Part model, mm, in its own coordinate system. Face numbers are marked on the shaded views. A direction names the side the tool comes from. Coordinates: 2 decimals unless noted, no trailing zeros. Loops run counter-clockwise (first coordinate to the right, second up) from the corner with the lowest first, then second, coordinate; pieces in that order, holes last.
```python
from build123d import *

# Parameters (mm, degrees)
F0_W     = 20.32
F0_H     = 19.186653
F1_DEPTH = 2.26077
F2_W     = 4.396148
F2_H     = 12.7
F3_DEPTH = 12.18664


with BuildPart() as f1:
    # F0 (on Front) → F1 (new body)
    with BuildSketch(Plane.XZ):
        with Locations((-10.16, 11.454718)):
            Rectangle(F0_W, F0_H)
    extrude(amount=F1_DEPTH)

    # F2 (on face) → F3 (join)
    with BuildSketch(Plane.XZ.offset(2.26077)):
        with Locations((-15.614839, 11.398978)):
            Rectangle(F2_W, F2_H)
        with Locations((-4.54603, 11.398978)):
            Rectangle(F2_W, F2_H)
    extrude(amount=F3_DEPTH)


solid = f1.part
```
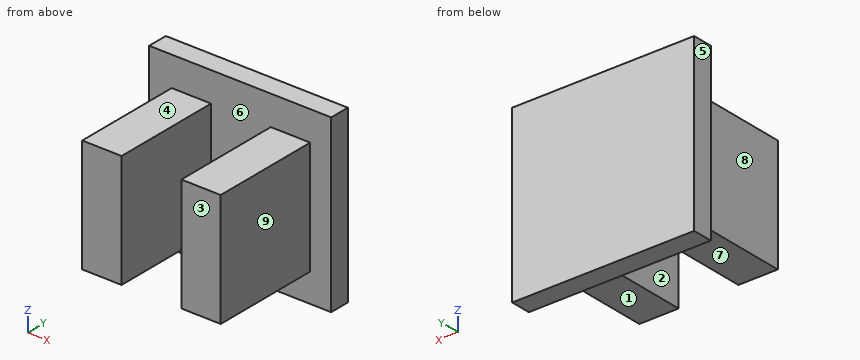
Q1. Tool access for the marked faces 1, 2, 3, 4 and 5: list every direction of +Z, -Z, +X, -X, +Y, -Y with a clear straight run to the whole face (end or side of a thin tool).
Q2. Mould opens along X. For the marked faces 6, 7, 8 and 9 say: released by +X, released by -X, zero draft, split by the parting line, or undercut.
Q3. Saw through at A-A (y = -11.25). List the corners of the cut face in (x, z).
Q4. Saw through at C-C (z = 14.5). List the corners of the cut face in (x, y), plus the area to 3 significant figures.
Q5. Probe line 1 (X direction, y = -12, z = 13.5); line 2 (Y direction, x = -12, z = 12.25); line 3 (Z direction, x = -4.75, y = -7.5). List the from-to ranges inside material, lowest first.
Q6. Saw through at D-D (z = 3.75). List the corners of the cut face in (x, y).
Q7. Saw through at B-B (x = -15.5). List the corners of the cut face in (y, z), plus the area to 3 significant figures.
Q8. Drop flat-ended pins along their axis: P1, Ø10, axis at x = -12, z = 4, coming from the -Y side; P2, Ø5, axis at x = -5, y = -10.5, coming from the -Z side; P3, Ø2, axis at y = -12, z = 7, coming from the +X side; P4, Ø2, axis at x = -16.5, y = -9.5, coming from the +Z side. Give the stop position or say it passes through.
Checked values:
1. face 1: -Z, +X, -X, -Y
1. face 2: +Z, -Z, -Y
1. face 3: +Z, -Z, +X, -X, -Y
1. face 4: +Z, +X, -X, -Y
1. face 5: +Z, -Z, -X, +Y, -Y
2. face 6: undercut
2. face 7: zero draft
2. face 8: released by -X
2. face 9: released by +X
3. outline: (-17.81, 5.05) - (-13.42, 5.05) - (-13.42, 17.75) - (-17.81, 17.75) - close; (-6.74, 5.05) - (-2.35, 5.05) - (-2.35, 17.75) - (-6.74, 17.75) - close
4. outline: (-20.32, -2.26) - (-17.81, -2.26) - (-17.81, -14.45) - (-13.42, -14.45) - (-13.42, -2.26) - (-6.74, -2.26) - (-6.74, -14.45) - (-2.35, -14.45) - (-2.35, -2.26) - (0, -2.26) - (0, 0) - (-20.32, 0) - close
4. area: 153 mm2
5. line 1: x = -17.81 to -13.42, -6.74 to -2.35
5. line 2: y = -2.26 to 0
5. line 3: z = 5.05 to 17.75
6. outline: (-20.32, -2.26) - (0, -2.26) - (0, 0) - (-20.32, 0) - close
7. outline: (-14.45, 5.05) - (-2.26, 5.05) - (-2.26, 1.86) - (0, 1.86) - (0, 21.05) - (-2.26, 21.05) - (-2.26, 17.75) - (-14.45, 17.75) - close
7. area: 198 mm2
8. P1: stops at y = -14.45
8. P2: stops at z = 5.05
8. P3: stops at x = -2.35
8. P4: stops at z = 17.75
